Can you work these out from the model? Positions are in its coordinate system, mm. A direction names the side the tool comes from. Coordinates: 2 decimals unless noted, no trailing zeros. Order: outer loops, then holes, each group sorted by start corner. A loop starts at its lowest first (then second) coordinate and runs counter-clockwise, first axis right, second up. Notation, with made-up numbers: (48.5, -5) -> (73.5, -5) arc R20 ccw to (73.5, 3) -> close; hole circle Ø1 at (-30.5, -21.75). An arc over 180 degrees is marked (long way). Answer in a Markdown table with one row per item.
```python
from build123d import *

# Parameters (mm, degrees)
CROQUIS1_W              = 72
CROQUIS1_H              = 180
CROQUIS1_R              = 2.85
CROQUIS1_R_2            = 1.5
SALIENTE_EXTRUIR1_DEPTH = 4
CROQUIS2_R              = 2.85
CORTAR_EXTRUIR1_DEPTH   = 1.65
CROQUIS3_W              = 4
CROQUIS3_H              = 10
SALIENTE_EXTRUIR2_DEPTH = 10
CORTAR_EXTRUIR2_REACH   = 263.951
CROQUIS4_R              = 1.5
CROQUIS4_3_R            = 1.5
CORTAR_EXTRUIR3_DEPTH   = 1.65
REDONDEO3_R             = 10
CROQUIS5_W              = 4
CROQUIS5_H              = 80
SALIENTE_EXTRUIR3_DEPTH = 50
SALIENTE_EXTRUIR4_DEPTH = 5
SALIENTE_EXTRUIR5_DEPTH = 5
CORTAR_EXTRUIR4_REACH   = 263.401
CROQUIS9_R              = 1.6


with BuildPart() as part:
    # Croquis1 → Saliente-Extruir1 (new body)
    # profile 1 of 5: a face of its own
    with BuildSketch(Plane.XY):
        with Locations((32, 162.773389683)):
            Rectangle(CROQUIS1_W, CROQUIS1_H)
        with Locations((4.48, 83.573389683)):
            Circle(CROQUIS1_R, mode=Mode.SUBTRACT)
        with Locations((11.52, 76.973389683)):
            Circle(CROQUIS1_R, mode=Mode.SUBTRACT)
        with Locations((11.52, 241.973389683)):
            Circle(CROQUIS1_R, mode=Mode.SUBTRACT)
        with Locations((4.48, 248.573389683)):
            Circle(CROQUIS1_R, mode=Mode.SUBTRACT)
    # profile 2 of 5: a face of its own
    with BuildSketch(Plane.XY):
        with Locations((4.48, 83.573389683)):
            Circle(CROQUIS1_R)
        with Locations((4.48, 83.573389683)):
            Circle(CROQUIS1_R_2, mode=Mode.SUBTRACT)
    # profile 3 of 5: a face of its own
    with BuildSketch(Plane.XY):
        with Locations((11.52, 76.973389683)):
            Circle(CROQUIS1_R)
        with Locations((11.52, 76.973389683)):
            Circle(CROQUIS1_R_2, mode=Mode.SUBTRACT)
    # profile 4 of 5: a face of its own
    with BuildSketch(Plane.XY):
        with Locations((11.52, 241.973389683)):
            Circle(CROQUIS1_R)
        with Locations((11.52, 241.973389683)):
            Circle(CROQUIS1_R_2, mode=Mode.SUBTRACT)
    # profile 5 of 5: a face of its own
    with BuildSketch(Plane.XY):
        with Locations((4.48, 248.573389683)):
            Circle(CROQUIS1_R)
        with Locations((4.48, 248.573389683)):
            Circle(CROQUIS1_R_2, mode=Mode.SUBTRACT)
    extrude(amount=SALIENTE_EXTRUIR1_DEPTH)

    # Croquis2 → Cortar-Extruir1 (cut)
    with BuildSketch(Plane.XY.offset(4)):
        with Locations((4.48, 248.573389683)):
            Circle(CROQUIS2_R)
        with Locations((11.52, 241.973389683)):
            Circle(CROQUIS2_R)
        with Locations((4.48, 83.573389683)):
            Circle(CROQUIS2_R)
        with Locations((11.52, 76.973389683)):
            Circle(CROQUIS2_R)
    extrude(amount=-CORTAR_EXTRUIR1_DEPTH, mode=Mode.SUBTRACT)

    # Croquis3 → Saliente-Extruir2 (add)
    with BuildSketch(Plane(origin=(0, 0, 0), x_dir=(-1, 0, 0), z_dir=(0, 0, -1))):
        with Locations((-2, 200.273389683)):
            Rectangle(CROQUIS3_W, CROQUIS3_H)
        with Locations((-2, 125.273389683)):
            Rectangle(CROQUIS3_W, CROQUIS3_H)
    extrude(amount=SALIENTE_EXTRUIR2_DEPTH)

    # Croquis4 → Cortar-Extruir2 (cut, up to next)
    with BuildSketch(Plane.ZY, mode=Mode.PRIVATE) as cortar_extruir2_sk1:
        with Locations(Location((-5, 125.273389683, 0), (0, 0, 270))):
            Circle(CROQUIS4_R)
    cortar_extruir2_tool1 = extrude(cortar_extruir2_sk1.sketch, amount=-CORTAR_EXTRUIR2_REACH, mode=Mode.PRIVATE) & part.part
    # Croquis4 → Cortar-Extruir2 (cut, up to next)
    with BuildSketch(Plane.ZY, mode=Mode.PRIVATE) as cortar_extruir2_sk2:
        with Locations(Location((-5, 200.273389683, 0), (0, 0, 270))):
            Circle(CROQUIS4_R)
    cortar_extruir2_tool2 = extrude(cortar_extruir2_sk2.sketch, amount=-CORTAR_EXTRUIR2_REACH, mode=Mode.PRIVATE) & part.part
    add(cortar_extruir2_tool1.solids().sort_by_distance((0, 125.27339, -5))[0], mode=Mode.SUBTRACT)
    add(cortar_extruir2_tool2.solids().sort_by_distance((0, 200.27339, -5))[0], mode=Mode.SUBTRACT)

    # Croquis4<3> → Cortar-Extruir3 (cut)
    # profile 1 of 2: a face of its own
    with BuildSketch(Plane.ZY):
        Polygon((-8.348631561, 200.273389683), (-6.674315781, 197.373389683), (-3.325684219, 197.373389683), (-1.651368439, 200.273389683), (-3.325684219, 203.173389683), (-6.674315781, 203.173389683), align=None)
        with Locations(Location((-5, 200.273389683, 0), (0, 0, 270))):
            Circle(CROQUIS4_3_R, mode=Mode.SUBTRACT)
    # profile 2 of 2: a face of its own
    with BuildSketch(Plane.ZY):
        Polygon((-8.348631561, 125.273389683), (-6.674315781, 122.373389683), (-3.325684219, 122.373389683), (-1.651368439, 125.273389683), (-3.325684219, 128.173389683), (-6.674315781, 128.173389683), align=None)
        with Locations(Location((-5, 125.273389683, 0), (0, 0, 270))):
            Circle(CROQUIS4_3_R, mode=Mode.SUBTRACT)
    extrude(amount=-CORTAR_EXTRUIR3_DEPTH, mode=Mode.SUBTRACT)

    # Redondeo3
    # the kernel refuses this fillet: 10 mm, written as the material it takes off along each edge
    with BuildSketch(Plane(origin=(68, 52.773389683, 4), x_dir=(0, 0, -1), z_dir=(0, 1, 0))) as redondeo3_piece_1:
        with BuildLine():
            CenterArc((10, 8), REDONDEO3_R, 180, 53.130102354)
            Line((0, 8), (-0.2, 8))
            Line((-0.2, 8), (-0.2, 0))
            Line((-0.2, 0), (0, -0.2))
            ThreePointArc((0, -0.2), (2, -0.2), (3.88, -0.16))
            Line((3.88, -0.16), (4, 0))
        make_face()
    extrude(amount=220, mode=Mode.SUBTRACT)

    # Croquis5 → Saliente-Extruir3 (add)
    with BuildSketch(Plane(origin=(0, 0, 0), x_dir=(-1, 0, 0), z_dir=(0, 0, -1))):
        with Locations((-26, 162.773389683)):
            Rectangle(CROQUIS5_W, CROQUIS5_H)
    extrude(amount=SALIENTE_EXTRUIR3_DEPTH)

    # Croquis6 → Saliente-Extruir4 (add)
    with BuildSketch(Plane(origin=(0, 202.773389683, 0), x_dir=(1, 0, 0), z_dir=(0, 1, 0))):
        Polygon((28, 0), (33, 0), (28, 10), align=None)
    extrude(amount=-SALIENTE_EXTRUIR4_DEPTH)

    # Croquis7 → Saliente-Extruir5 (add)
    with BuildSketch(Plane.XZ.offset(-122.773389683)):
        Polygon((28, 0), (33, 0), (28, -10), align=None)
    extrude(amount=-SALIENTE_EXTRUIR5_DEPTH)

    # Croquis9 → Cortar-Extruir4 (cut, up to next)
    with BuildSketch(Plane.ZY.offset(-24), mode=Mode.PRIVATE) as cortar_extruir4_sk1:
        with Locations(Location((-9, 191.273389683, 0), (0, 0, 270))):
            Circle(CROQUIS9_R)
    cortar_extruir4_tool1 = extrude(cortar_extruir4_sk1.sketch, amount=-CORTAR_EXTRUIR4_REACH, mode=Mode.PRIVATE) & part.part
    # Croquis9 → Cortar-Extruir4 (cut, up to next)
    with BuildSketch(Plane.ZY.offset(-24), mode=Mode.PRIVATE) as cortar_extruir4_sk2:
        with Locations(Location((-41, 191.273389683, 0), (0, 0, 270))):
            Circle(CROQUIS9_R)
    cortar_extruir4_tool2 = extrude(cortar_extruir4_sk2.sketch, amount=-CORTAR_EXTRUIR4_REACH, mode=Mode.PRIVATE) & part.part
    # Croquis9 → Cortar-Extruir4 (cut, up to next)
    with BuildSketch(Plane.ZY.offset(-24), mode=Mode.PRIVATE) as cortar_extruir4_sk3:
        with Locations(Location((-41, 134.273389683, 0), (0, 0, 270))):
            Circle(CROQUIS9_R)
    cortar_extruir4_tool3 = extrude(cortar_extruir4_sk3.sketch, amount=-CORTAR_EXTRUIR4_REACH, mode=Mode.PRIVATE) & part.part
    # Croquis9 → Cortar-Extruir4 (cut, up to next)
    with BuildSketch(Plane.ZY.offset(-24), mode=Mode.PRIVATE) as cortar_extruir4_sk4:
        with Locations(Location((-9, 134.273389683, 0), (0, 0, 270))):
            Circle(CROQUIS9_R)
    cortar_extruir4_tool4 = extrude(cortar_extruir4_sk4.sketch, amount=-CORTAR_EXTRUIR4_REACH, mode=Mode.PRIVATE) & part.part
    add(cortar_extruir4_tool1.solids().sort_by_distance((24, 191.27339, -9))[0], mode=Mode.SUBTRACT)
    add(cortar_extruir4_tool2.solids().sort_by_distance((24, 191.27339, -41))[0], mode=Mode.SUBTRACT)
    add(cortar_extruir4_tool3.solids().sort_by_distance((24, 134.27339, -41))[0], mode=Mode.SUBTRACT)
    add(cortar_extruir4_tool4.solids().sort_by_distance((24, 134.27339, -9))[0], mode=Mode.SUBTRACT)


solid = part.part
```
(1) Suppose I cut it at A-A (y = 139.5). Please give me the cut outline in (x, z), and give its area (3 significant figures).
Response values:
| item | result |
|---|---|
| outline | (-4, 0) -> (24, 0) -> (24, -50) -> (28, -50) -> (28, 0) -> (68, 0) arc R10 ccw to (60, 4) -> (-4, 4) -> close |
| area | 478 mm2 |
(2) On a 3-axis mill with a long thin cutter (end or side, diameter ignored), from which of +Z, -Z, +X, -X, +Y, -Y can I reach the whole of each face in a straight line? I mean faces 1 (the flat face through (2, 205.273, -5)), 2 (the flat face through (0, 202.4, -2.7)), 3 (the flat face through (1.65, 127, -4)), 4 (the flat face through (13, 241, 2.35)), 5 (the flat face through (4, 124.1, -3.8)). Say none if no direction works.
Response values:
| item | result |
|---|---|
| face 1 | -Z, +X, -X, +Y |
| face 2 | -Z, -X, +Y, -Y |
| face 3 | -X |
| face 4 | +Z |
| face 5 | -Z, +Y, -Y |
(3) Will these pins go through, and if not, where does the flat tip stop? pin 1 Ø1.5 at (x, y) = (60.5, 142) entering from -Z; pin 2 Ø4.5 at (x, z) = (1, -5) entering from +Y; pin 3 Ø12 at (y, z) = (174, -8.5) entering from -X.
Response values:
| item | result |
|---|---|
| pin 1 | z = 0 |
| pin 2 | y = 205.27 |
| pin 3 | x = 24 |
(4) Suppose I cut it at B-B (x = 56). Please give me the cut outline in (y, z), and give its area (3 significant figures).
Response values:
| item | result |
|---|---|
| outline | (72.77, 0) -> (252.77, 0) -> (252.77, 4) -> (72.77, 4) -> close |
| area | 720 mm2 |
(5) We'd pull the mould along Z, two halves only. Please class faces 6 (the flat face through (2, 125, -10)), 7 (the cylindrical face through (25.972, 189.795, -9.613)), 8 (the cylindrical face through (12.835, 239.445, 3.187)): +Z half, -Z half, draft (parallel to the pull), parting line (faces both ways), or undercut.
Response values:
| item | result |
|---|---|
| face 6 | -Z half |
| face 7 | undercut |
| face 8 | draft |
(6) I need wall thicknesses on line 1 (Z direction, x = 48, y = 149); line 2 (X direction, y = 197, z = -37); line 3 (X direction, y = 203, z = -6.5). Which ranges of each line are inside material? Lowest first, please. Write a range as [from, to].
Response values:
| item | result |
|---|---|
| line 1 | [0, 4] |
| line 2 | [24, 28] |
| line 3 | [1.65, 4] |
(7) Suppose I cut it at C-C (z = -22). Please give me the cut outline in (x, y), and give its area (3 significant figures).
Response values:
| item | result |
|---|---|
| outline | (24, 122.77) -> (28, 122.77) -> (28, 202.77) -> (24, 202.77) -> close |
| area | 320 mm2 |
